from build123d import *

# Parameters (mm, degrees)
SKETCH2_W           = 40
SKETCH2_H           = 12.7
BOSS_EXTRUDE1_DEPTH = 6.35
SKETCH3_W           = 27.3
SKETCH3_H           = 6.35
BOSS_EXTRUDE2_DEPTH = 12.7
SKETCH4_W           = 4.9
SKETCH4_H           = 6.35
CUT_EXTRUDE1_DEPTH  = 8.6


with BuildPart() as part:
    # Sketch2 → Boss-Extrude1 (new body)
    with BuildSketch(Plane.XY):
        Rectangle(SKETCH2_W, SKETCH2_H)
    extrude(amount=BOSS_EXTRUDE1_DEPTH)

    # Sketch3 → Boss-Extrude2 (add)
    with BuildSketch(Plane.XZ.offset(6.35)):
        with Locations((0, 3.175)):
            Rectangle(SKETCH3_W, SKETCH3_H)
    extrude(amount=BOSS_EXTRUDE2_DEPTH)

    # Sketch4 → Cut-Extrude1 (cut)
    with BuildSketch(Plane(origin=(0, 6.35, 0), x_dir=(1, 0, 0), z_dir=(0, 1, 0))):
        with Locations((0, -3.175)):
            Rectangle(SKETCH4_W, SKETCH4_H)
    extrude(amount=-CUT_EXTRUDE1_DEPTH, mode=Mode.SUBTRACT)


solid = part.part
CAD build for the part. Positions are in the model's coordinates, mm. A direction names the side the tool comes from. Coordinates: 2 decimals unless noted, no trailing zeros. Write each loop counter-clockwise with the first axis right and the second up, starting at its lowest first coordinate (ties: lowest second). Pieces come first, ordered by that corner, then holes. Notation, with made-up numbers: M 47.5,9 L 76.5,9 A12 ccw 76.5,32 Z; hole C -0.5,45.5 d11. An arc over 180 degrees is marked long. Return JSON: item names as keys, results as strings.
Item 1: Probe line 1 (X direction, y = 5, z = 2); line 2 (Y direction, x = -0.5, z = 4); line 3 (X direction, y = -10.75, z = 1.5). List the from-to ranges inside material, lowest first. Write a range as from..to.
Findings below:
{"line 1": "x = -20..-2.45, 2.45..20", "line 2": "y = -19.05..-2.25", "line 3": "x = -13.65..13.65"}
Item 2: Slice it at C-C, the plane x = 15.5. Write the cut outline in (y, z), and give its area (3 significant figures).
Findings below:
{"outline": "M -6.35,0 L 6.35,0 L 6.35,6.35 L -6.35,6.35 Z", "area": "80.6 mm2"}
Item 3: Slice it at D-D, the plane y = -15. Write the cut outline in (x, z).
Findings below:
{"outline": "M -13.65,0 L 13.65,0 L 13.65,6.35 L -13.65,6.35 Z"}
Item 4: Slice it at A-A, the plane y = -0.25. Write the cut outline in (x, z).
Findings below:
{"outline": "M -20,0 L -2.45,0 L -2.45,6.35 L -20,6.35 Z; M 2.45,0 L 20,0 L 20,6.35 L 2.45,6.35 Z"}
Item 5: Slice it at B-B, the plane z = 3.25. Write the cut outline in (x, y).
Findings below:
{"outline": "M -20,-6.35 L -13.65,-6.35 L -13.65,-19.05 L 13.65,-19.05 L 13.65,-6.35 L 20,-6.35 L 20,6.35 L 2.45,6.35 L 2.45,-2.25 L -2.45,-2.25 L -2.45,6.35 L -20,6.35 Z"}
Item 6: Two-plate mould, pull along X, no slides. Class faces 1 (the flat face through (0, -2.25, 3)), 2 (the flat face through (13.65, -13, 3)), 3 (the flat face through (11, 6.35, 3)), 4 (the flat face through (-2.45, 2, 3)): +X half, -X half, draft (parallel to the pull), parting line (faces both ways), or undercut.
Findings below:
{"face 1": "undercut", "face 2": "+X half", "face 3": "draft", "face 4": "undercut"}
Item 7: Drop flat-ended pins along their axis: pin 1 Ø3 at (x, y) = (14.5, -0.5) entering from -Z; pin 2 Ø1.5 at (y, z) = (-13, 2) entering from +X; pin 3 Ø1.9 at (y, z) = (-11.5, 1.5) entering from -X. Give the stop position or say it passes through.
Findings below:
{"pin 1": "stops at z = 0", "pin 2": "stops at x = 13.65", "pin 3": "stops at x = -13.65"}
Item 8: Which spindle directions (+Z, -Z, +X, -X, +Y, -Y) get a long thin tool onto all of the face, cutting with end or side? Do faces 5 (the flat face through (-20, 0, 3)), 6 (the flat face through (2.45, 2, 3)), 7 (the flat face through (17, -6.35, 3)), 8 (the flat face through (0, -6, 0)), 9 (the flat face through (-13.65, -13, 3)). Say none if no direction does.
Findings below:
{"face 5": "+Z, -Z, -X, +Y, -Y", "face 6": "+Z, -Z, +Y", "face 7": "+Z, -Z, +X, -Y", "face 8": "-Z, +X, -X, +Y, -Y", "face 9": "+Z, -Z, -X, -Y"}
